```python
from build123d import *

# Parameters (mm, degrees)
CBORE_FOR_M3_HEX_HEAD_BOLT1_D           = 3.4
CBORE_FOR_M3_HEX_HEAD_BOLT1_CBORE_D     = 6
CBORE_FOR_M3_HEX_HEAD_BOLT1_CBORE_DEPTH = 35
CUT_EXTRUDE1_DEPTH                      = 43.521318352
CUT_EXTRUDE1_DEPTH_BACK                 = 43.521318352
SKETCH1_W                               = 45.460757026
SKETCH1_H                               = 38.1
CUT_EXTRUDE2_DEPTH                      = 3.96875
SKETCH3_R                               = 6.985
CUT_EXTRUDE3_DEPTH                      = 1.27
SKETCH4_R                               = 3.96875
CUT_EXTRUDE4_DEPTH                      = 30.601262411


with BuildPart() as part:
    # 草图1 → 旋转1 (revolve)
    with BuildSketch(Plane.XY):
        with BuildLine():
            Line((0, 0), (0, 31.75))
            Line((0, 31.75), (5.477501396, 31.75))
            add(Edge.make_bspline(
                [(5.477501396, 31.75), (16.24161295, 23.874290145), (19.406701728, 11.219456234), (20, 0)],
                knots=[0.132414506, 0.132414506, 0.132414506, 0.132414506, 1, 1, 1, 1], degree=3))
            Line((20, 0), (0, 0))
        make_face()
    revolve(axis=Axis((0, 0, 0), (0, 1, 0)))

    # CBORE for M3 Hex Head Bolt1 (through all)
    with Locations(Plane(origin=(0, 40, 0), x_dir=(-1, 0, 0), z_dir=(0, 1, 0))):
        with Locations((0, -9.525), (0, 9.525)):
            CounterBoreHole(CBORE_FOR_M3_HEX_HEAD_BOLT1_D / 2, CBORE_FOR_M3_HEX_HEAD_BOLT1_CBORE_D / 2, CBORE_FOR_M3_HEX_HEAD_BOLT1_CBORE_DEPTH)

    # Sketch1 → Cut-Extrude1 (cut, two sides: drawn at the far end of the back side and taken through both)
    with BuildSketch(Plane.XY.offset(-CUT_EXTRUDE1_DEPTH_BACK)):
        with Locations((0, 31.75)):
            Rectangle(SKETCH1_W, SKETCH1_H)
    extrude(amount=CUT_EXTRUDE1_DEPTH + CUT_EXTRUDE1_DEPTH_BACK, mode=Mode.SUBTRACT)

    # Sketch2 → Cut-Extrude2 (cut)
    with BuildSketch(Plane(origin=(0, 12.7, 0), x_dir=(1, 0, 0), z_dir=(0, 1, 0))):
        with BuildLine():
            Line((-3, 9.525), (-3, 5.596650784))
            ThreePointArc((-3, 5.596650784), (-6.35, 0), (-3, -5.596650784))
            Line((-3, -5.596650784), (-3, -9.525))
            ThreePointArc((-3, -9.525), (0, -12.525), (3, -9.525))
            Line((3, -9.525), (3, -5.596650784))
            ThreePointArc((3, -5.596650784), (6.35, 0), (3, 5.596650784))
            Line((3, 5.596650784), (3, 9.525))
            ThreePointArc((3, 9.525), (0, 12.525), (-3, 9.525))
        make_face()
    extrude(amount=-CUT_EXTRUDE2_DEPTH, mode=Mode.SUBTRACT)

    # Sketch3 → Cut-Extrude3 (cut)
    with BuildSketch(Plane(origin=(0, 12.7, 0), x_dir=(1, 0, 0), z_dir=(0, 1, 0))):
        Circle(SKETCH3_R)
    extrude(amount=-CUT_EXTRUDE3_DEPTH, mode=Mode.SUBTRACT)

    # Sketch4 → Cut-Extrude4 (cut, through all)
    with BuildSketch(Plane(origin=(0, 8.73125, 0), x_dir=(1, 0, 0), z_dir=(0, 1, 0))):
        with Locations(Location((0, 0, 0), (0, 0, 270))):
            Circle(SKETCH4_R)
    extrude(amount=-CUT_EXTRUDE4_DEPTH, mode=Mode.SUBTRACT)


solid = part.part
```
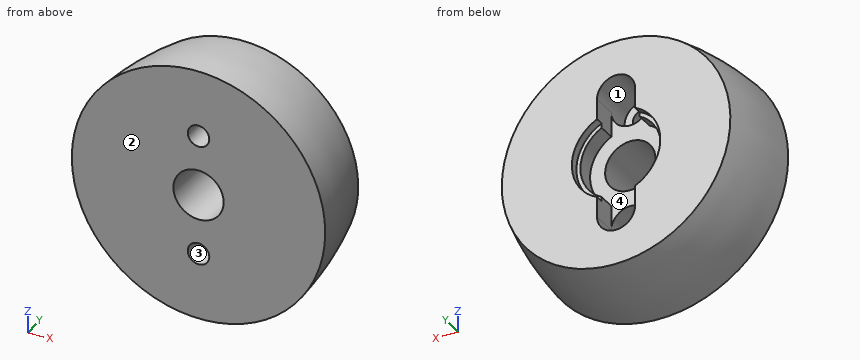
CAD build for the part. Positions are in the model's coordinates, mm. Face numbers are marked on the shaded views. A direction names the side the tool comes from. Give positions to 0.01 mm unless a question says otherwise; leave off trailing zeros. Put each result on its own line as item: value.
Q1. Tool access for the marked faces 3 and 4: list every direction of +Z, -Z, +X, -X, +Y, -Y with a clear straight run to the whole face (end or side of a thin tool).
Filled in:
face 3: +Y, -Y
face 4: +Y
Q2. Mould opens along X. For the marked faces 1 and 2 say: pulls with the +X half, pulls with the -X half, needs draft (parallel to the pull), parting line crosses it, or undercut.
Filled in:
face 1: undercut
face 2: needs draft
Q3. Probe line 1 along Y through (x, z) = (-2.5, 10); line 2 along Z through (x, y) = (5, 12); line 3 along Z through (x, y) = (-2.5, 4.5). List the from-to ranges inside material, lowest first.
Filled in:
line 1: y = 0 to 5
line 2: z = -17.53 to -4.88, 4.88 to 17.53
line 3: z = -19.46 to -3.08, 3.08 to 19.46
Q4. Slice it at A-A (x = 0). Give the number of separate pieces and of enclosed holes in the cut face, plus the area to 3 significant figures.
Filled in:
separate pieces: 4
enclosed holes: 0
area: 242 mm²
Q5. Flat gauge pins, fed straight in: pin 1 (6 mm diameter, centred on y = 11, z = 10, fed in from +X); pin 2 (5 mm diameter, centred on y = 10.5, z = 16, fed in from +X); pin 3 (2 mm diameter, centred on x = 4, z = -3, fed in from +Y); pin 4 (5 mm diameter, centred on x = 0, z = 9.525, fed in from -Y). Where does each tip first touch, or does it go through?
Filled in:
pin 1: stops at x = 17.3
pin 2: stops at x = 12.91
pin 3: stops at y = 8.73
pin 4: stops at y = 0
